from build123d import *

# Parameters (mm, degrees)
BOSS_EXTRU_1_DEPTH      = 8
TROU_TARAUD_M51_D       = 4.2
TROU_TARAUD_M52_D       = 4.2
ESQUISSE8_W             = 18.974951104
ESQUISSE8_H             = 96.168502187
ENL_V_MAT_EXTRU_1_DEPTH = 34


with BuildPart() as part:
    # Esquisse1 → Boss.-Extru.1 (new body)
    with BuildSketch(Plane.XY):
        with BuildLine():
            Line((-202.4, -38.343708741), (-202.4, -50))
            Line((-202.4, -50), (-206.431005423, -50))
            ThreePointArc((-206.431005423, -50), (-212.4, 0), (-206.431005423, 50))
            Line((-206.431005423, 50), (-202.4, 50))
            Line((-202.4, 50), (-202.4, 38.343708741))
            ThreePointArc((-202.4, 38.343708741), (-206, 0), (-202.4, -38.343708741))
        make_face()
    extrude(amount=BOSS_EXTRU_1_DEPTH)

    # Trou taraudé M51 (through all)
    with Locations(Plane(origin=(-202.4, 0, 0), x_dir=(0, 0, -1), z_dir=(1, 0, 0))):
        with Locations((-4, 35)):
            Hole(TROU_TARAUD_M51_D / 2)

    # Trou taraudé M52 (through all)
    with Locations(Plane(origin=(-202.4, 0, 0), x_dir=(0, 0, -1), z_dir=(1, 0, 0))):
        with Locations((-4, -35)):
            Hole(TROU_TARAUD_M52_D / 2)

    # Esquisse8 → Enlèv. mat.-Extru.1 (cut)
    with BuildSketch(Plane.XY):
        with Locations((-220.887475552, -0.394191452)):
            Rectangle(ESQUISSE8_W, ESQUISSE8_H)
    extrude(amount=ENL_V_MAT_EXTRU_1_DEPTH, mode=Mode.SUBTRACT)


solid = part.part
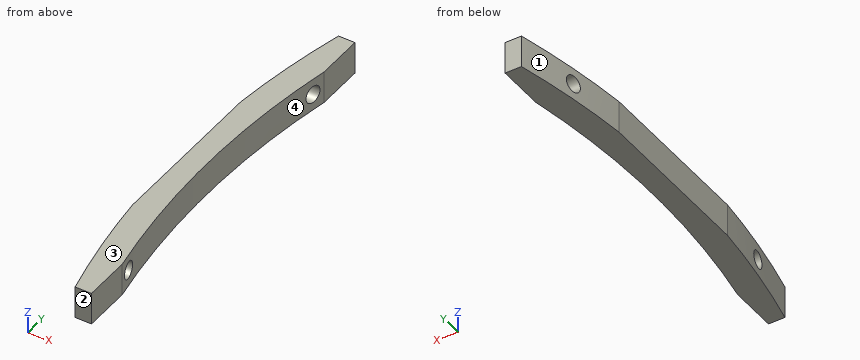
The listing builds one solid part. Answer for the finished solid, in the listing's coordinates (mm). Face numbers are marked on the shaded views. Coordinates: 2 decimals unless noted, no trailing zeros. Loops run counter-clockwise (first coordinate to the right, second up) from the corner with the lowest first, then second, coordinate; pieces in that order, holes last.
1) Determine the mould class of the marked faces 1, 2, 3 and 4 for opening direction Y: pulls with the +Y half, pulls with the -Y half, needs draft (parallel to the pull), parting line crosses it, or undercut.
2) Find the intervals of material crossed by L1, parallel to Z at x = -204.25, y = -35; L2, parallel to X at y = -1, z = 4.75; L3, parallel to X at y = 33.5, z = 5.5, in increasing order.
3) Find section A-A on x = -205. Write down the section's boundary in (y, z).
4) Find section D-D on y = 17.5. Write down the section's boundary in (x, z), then the cut area to 3 significant figures.
5) Find section C-C on z = 4. Write down the section's boundary in (x, y).
6) Find section B-B on y = -35. Write down the section's boundary in (x, z).
Values:
1. face 1: pulls with the +Y half
1. face 2: pulls with the -Y half
1. face 3: needs draft
1. face 4: undercut
2. L1: z = 0 to 1.9, 6.1 to 8
2. L2: x = -211.4 to -206
2. L3: x = -209.74 to -203.26
3. outline: (-50, 0) - (-20.27, 0) - (-20.27, 8) - (-50, 8) - close; (20.27, 0) - (50, 0) - (50, 8) - (20.27, 8) - close; hole circle Ø4.2 at (-35, 4); hole circle Ø4.2 at (35, 4)
4. outline: (-211.4, 0) - (-205.26, 0) - (-205.26, 8) - (-211.4, 8) - close
4. area: 49.2 mm2
5. outline: (-211.4, -20.59) arc R212.4 ccw to (-209.84, -32.9) - (-203.36, -32.9) arc R206 cw to (-203.36, 32.9) - (-209.84, 32.9) arc R212.4 ccw to (-211.4, 20.59) - close; (-209.13, -37.1) arc R212.4 ccw to (-206.43, -50) - (-202.4, -50) - (-202.4, -38.34) arc R206 cw to (-202.63, -37.1) - close; (-209.13, 37.1) - (-202.63, 37.1) arc R206 cw to (-202.4, 38.34) - (-202.4, 50) - (-206.43, 50) arc R212.4 ccw to start
6. outline: (-209.5, 0) - (-203, 0) - (-203, 1.9) - (-209.5, 1.9) - close; (-209.5, 6.1) - (-203, 6.1) - (-203, 8) - (-209.5, 8) - close
